Design review of the part built by this model. Coordinates are the model's own, in mm. Round coordinates to 2 decimals unless told otherwise and drop trailing zeros. Loops run counter-clockwise (first coordinate to the right, second up) from the corner with the lowest first, then second, coordinate; pieces in that order, holes last. Notation, with made-up numbers: (-26, -28) -> (15, -28) arc R24 ccw to (15, -3) -> close; hole circle Ø9 at (41, 29.5). An arc over 180 degrees is marked (long way). Answer as CSV lines item,"result". Start each with the question number.
(1) For P1, Ø2, axis at y = -37, z = 26, coming from the +X side; P2, Ø5, axis at y = -53.5, z = 26.5, coming from the +X side; P3, Ø3, axis at y = -71.5, z = 30.5, coming from the +X side, all flat-tipped, find the tip position at first contact; note any pin that passes through.
(2) Take a section at B-B, the plane y = -43. Write out the cut boundary in (x, z), and give its area (3 significant figures).
(3) Take a section at D-D, the plane x = 89. Write out the cut boundary in (y, z), and give its area (3 significant figures).
(4) Take a section at A-A, the plane z = 47.5. Write out the cut boundary in (x, y).
(5) To check wall thickness, follow line 1 (X direction, y = -43, z = 34); line 2 (Y direction, x = 87, z = 68); line 3 (X direction, y = -37.5, z = 10.5). State the ranges of each line that lie inside material, in increasing order. Write a range as from..to.
(6) Take a section at C-C, the plane z = 7.5. Write out the cut boundary in (x, y).
from build123d import *

# Parameters (mm, degrees)
F0_W     = 279.4
F0_H     = 76.2
F1_DEPTH = 76.2
F3_DEPTH = 76.201
F5_DEPTH = 76.201


with BuildPart() as f1:
    # F0 (on Top) → F1 (new body)
    with BuildSketch(Plane.XY):
        with Locations((-11.931214, -48.632389)):
            Rectangle(F0_W, F0_H)
    extrude(amount=F1_DEPTH)

    # F2 (on face) → F3 (cut, through all)
    with BuildSketch(Plane.XZ.offset(86.732389)):
        Polygon((127.768786, 0), (127.768786, 76.2), (77.787049, 0), align=None)
    extrude(amount=-F3_DEPTH, mode=Mode.SUBTRACT)

    # F4 (on face) → F5 (cut, through all)
    with BuildSketch(Plane.XY.offset(76.2)):
        Polygon((59.04955, -10.532389), (127.768786, -48.632389), (127.768786, -10.532389), align=None)
        Polygon((127.768786, -48.632389), (59.04955, -86.732389), (127.768786, -86.732389), align=None)
    extrude(amount=-F5_DEPTH, mode=Mode.SUBTRACT)


solid = f1.part
The answers:
1,P1,"x = 95.5"
1,P2,"x = 96.81"
1,P3,"x = 89.23"
2,outline,"(-151.63, 0) -> (77.79, 0) -> (117.61, 60.71) -> (117.61, 76.2) -> (-151.63, 76.2) -> close"
2,area,"19,300 mm²"
3,outline,"(-70.13, 17.09) -> (-27.14, 17.09) -> (-27.14, 76.2) -> (-70.13, 76.2) -> close"
3,area,"2,540 mm²"
4,outline,"(-151.63, -86.73) -> (59.05, -86.73) -> (108.94, -59.07) -> (108.94, -38.2) -> (59.05, -10.53) -> (-151.63, -10.53) -> close"
5,line 1,"-151.63..100.09"
5,line 2,"-71.24..-26.03"
5,line 3,"-151.63..84.67"
6,outline,"(-151.63, -86.73) -> (59.05, -86.73) -> (82.71, -73.62) -> (82.71, -23.65) -> (59.05, -10.53) -> (-151.63, -10.53) -> close"
